Work out the finished part from the listing and answer in its coordinate system (mm). A direction names the side the tool comes from. Give positions to 0.01 mm unless a question says otherwise; leave off trailing zeros. Loops run counter-clockwise (first coordinate to the right, second up) from the corner with the lowest first, then second, coordinate; pieces in that order, holes last. Notation, with made-up numbers: (20.25, 18.25) -> (75.25, 18.25) arc R23 ccw to (75.25, 43.25) -> close; hole circle Ø9 at (-6.5, 68). An arc over 180 degrees is marked (long way). Answer as CSV lines item,"result". Start each with the question number.
1. Determine the mould class of faces 1 (the face through (-27, 10.16, -8)), 2 (the face through (0, 7.302, 12)), 3 (the face through (7.296, 1.409, -7.956)), 4 (the face through (35.887, 5.009, -4.712)) for opening direction Z: +Z half, -Z half, draft (parallel to the pull), parting line (faces both ways), or undercut.
2. A tool of negligible diameter and unlimited length cuts with its end or side. For faces 5 (the face through (-5, 10.16, 5)), 6 (the face through (7.296, 8.751, -7.956)), 7 (the face through (-27.15, 1.41, -6.03)), from which of +Z, -Z, +X, -X, +Y, -Y can it reach the whole face along a straight path? Write none if from no direction.
3. Find section D-D, the plane x = -15.5. Give the vertices of the cut face in (y, z), and give its area (3 significant figures).
4. Find section C-C, the plane y = 5.25. Give the vertices of the cut face in (x, z) (3 decimals), and give its area (3 significant figures).
5. Find the intervals of material crossed by line 1 along X through (y, z) = (1.3, 0) (3 decimals); line 2 along Z through (x, y) = (9, 1.5); line 3 along Y through (x, z) = (17, -21.5), in increasing order.
6. Flat-ended cylindrical pins translate along their axes: pin 1 Ø3 at (y, z) = (7, 6.5) entering from +X; pin 2 Ø6 at (y, z) = (8, 14.5) entering from -X; pin 3 Ø3 at (x, y) = (23, 7.5) entering from -Z. Find the tip coordinate at first contact, or state that the pin passes through.
from build123d import *

# Parameters (mm, degrees)
SKETCH1_R          = 36.195
SKETCH1_R_2        = 6.35
DISK_DEPTH         = 10.16
SKETCH2_R          = 27.813
SKETCH2_R_2        = 10.795
CUT_EXTRUDE1_DEPTH = 2.8575


with BuildPart() as part:
    # Sketch1 → Disk (new body)
    with BuildSketch(Plane(origin=(0, 0, 0), x_dir=(1, 0, 0), z_dir=(0, 1, 0))):
        with Locations(Location((0, 0, 0), (0, 0, 270))):
            Circle(SKETCH1_R)
        with Locations(Location((0, 0, 0), (0, 0, 270))):
            Circle(SKETCH1_R_2, mode=Mode.SUBTRACT)
    extrude(amount=DISK_DEPTH)

    # Sketch2 → Cut-Extrude1 (cut)
    with BuildSketch(Plane(origin=(0, 10.16, 0), x_dir=(1, 0, 0), z_dir=(0, 1, 0))):
        with Locations(Location((0, 0, 0), (0, 0, 270))):
            Circle(SKETCH2_R)
        with Locations(Location((0, 0, 0), (0, 0, 270))):
            Circle(SKETCH2_R_2, mode=Mode.SUBTRACT)
    cut_extrude1 = extrude(amount=-CUT_EXTRUDE1_DEPTH, mode=Mode.SUBTRACT)

    # Mirror1: Cut-Extrude1 across plane
    add(cut_extrude1.mirror(Plane.ZX.offset(5.08)), mode=Mode.SUBTRACT)


solid = part.part
Resolved:
1,face 1,"draft"
1,face 2,"undercut"
1,face 3,"undercut"
1,face 4,"parting line"
2,face 5,"+Z, -Z, +X, -X, +Y"
2,face 6,"+Y"
2,face 7,"-Y"
3,outline,"(0, -32.71) -> (10.16, -32.71) -> (10.16, -23.09) -> (7.3, -23.09) -> (7.3, 23.09) -> (10.16, 23.09) -> (10.16, 32.71) -> (0, 32.71) -> (0, 23.09) -> (2.86, 23.09) -> (2.86, -23.09) -> (0, -23.09) -> close"
3,area,"401 mm^2"
4,outline,"circle Ø72.39 at (0, 0); hole circle Ø12.7 at (0, 0)"
4,area,"3,990 mm^2"
5,line 1,"x = -36.195 to -27.813, -10.795 to -6.35, 6.35 to 10.795, 27.813 to 36.195"
5,line 2,"z = -35.06 to -26.32, -5.96 to 5.96, 26.32 to 35.06"
5,line 3,"y = 2.86 to 7.3"
6,pin 1,"stops at x = 35.85"
6,pin 2,"stops at x = -34.32"
6,pin 3,"stops at z = -29.12"
